The listing builds one solid part. Answer for the finished solid, in the listing's coordinates (mm). A direction names the side the tool comes from. Give positions to 0.01 mm unless a question says otherwise; leave off trailing zeros. Write each loop counter-clockwise with the first axis right and the second up, starting at its lowest first coordinate (ties: lowest second). Pieces come first, ordered by that corner, then holes. Notation, with made-up numbers: (49, 85.5) - (103, 85.5) arc R18 ccw to (103, 120.5) - close; hole circle Ø3 at (84, -38). An arc over 180 degrees is marked (long way). Return JSON: item names as keys, results as strings.
from build123d import *

# Parameters (mm, degrees)
SKETCH1_W           = 1524
SKETCH1_H           = 762
BOSS_EXTRUDE1_DEPTH = 1016
SKETCH3_W           = 762
SKETCH3_H           = 507.878356785
CUT_EXTRUDE1_DEPTH  = 1016
CUT_EXTRUDE2_DEPTH  = 260.604
SKETCH6_W           = 254
SKETCH6_H           = 507.878356785
CUT_EXTRUDE3_DEPTH  = 1081.278
SKETCH7_W           = 254
SKETCH7_H           = 508
CUT_EXTRUDE4_DEPTH  = 1081.278
SKETCH8_W           = 508.045957887
SKETCH8_H           = 254
CUT_EXTRUDE5_DEPTH  = 1081.278
CUT_EXTRUDE6_DEPTH  = 835.406


with BuildPart() as part:
    # Sketch1 → Boss-Extrude1 (new body)
    with BuildSketch(Plane.XY):
        with Locations((-762, 381)):
            Rectangle(SKETCH1_W, SKETCH1_H)
    extrude(amount=BOSS_EXTRUDE1_DEPTH)

    # Sketch3 → Cut-Extrude1 (cut)
    with BuildSketch(Plane(origin=(0, 0, 0), x_dir=(-1, 0, 0), z_dir=(0, 0, -1))):
        with Locations((1143, 508.060821607)):
            Rectangle(SKETCH3_W, SKETCH3_H)
    extrude(amount=-CUT_EXTRUDE1_DEPTH, mode=Mode.SUBTRACT)

    # Sketch5 → Cut-Extrude2 (cut)
    with BuildSketch(Plane(origin=(0, 254.121643215, 0), x_dir=(1, 0, 0), z_dir=(0, 1, 0))):
        Polygon((-1524, -1016), (-762, 0), (-1524, 0), align=None)
    extrude(amount=-CUT_EXTRUDE2_DEPTH, mode=Mode.SUBTRACT)

    # Sketch6 → Cut-Extrude3 (cut)
    with BuildSketch(Plane.ZY.offset(762)):
        with Locations((127, 508.060821607)):
            Rectangle(SKETCH6_W, SKETCH6_H)
    extrude(amount=-CUT_EXTRUDE3_DEPTH, mode=Mode.SUBTRACT)

    # Sketch7 → Cut-Extrude4 (cut)
    with BuildSketch(Plane.ZY.offset(762)):
        with Locations((381, 508.121643215)):
            Rectangle(SKETCH7_W, SKETCH7_H)
    extrude(amount=-CUT_EXTRUDE4_DEPTH, mode=Mode.SUBTRACT)

    # Sketch8 → Cut-Extrude5 (cut)
    with BuildSketch(Plane(origin=(0, 254.121643215, 0), x_dir=(1, 0, 0), z_dir=(0, 1, 0))):
        with Locations((-254.022978944, -127)):
            Rectangle(SKETCH8_W, SKETCH8_H)
    extrude(amount=-CUT_EXTRUDE5_DEPTH, mode=Mode.SUBTRACT)

    # Sketch10 → Cut-Extrude6 (cut)
    with BuildSketch(Plane.ZY.offset(762)):
        Polygon((1016, 762), (508, 762), (508, 508.060821608), align=None)
    extrude(amount=-CUT_EXTRUDE6_DEPTH, mode=Mode.SUBTRACT)


solid = part.part
Item 1: Consider L1, parallel to X at y = 261.5, z = 706.5; L2, parallel to Y at x = -1258, z = 961; L3, parallel to Z at x = -301.5, y = 451. Determine where each line is inside the solid, lowest interval first.
Answer below:
{"L1": "x = -762 to 0", "L2": "y = 0 to 254.12", "L3": "z = 508 to 1016"}
Item 2: For faces 1 (the face through (-603, 0, 614)), 2 (the face through (-508.046, 129, 129)), 3 (the face through (-386, 379, 508)), 4 (the face through (-762, 448, 758)), 5 (the face through (-637, 129, 0)), determine the directions among +Z, -Z, +X, -X, +Y, -Y from which every point of the face is accessible in a straight line to the end or side of a thin tool.
Answer below:
{"face 1": "+Z, -Z, +X, -X, -Y", "face 2": "-Z, +X, +Y, -Y", "face 3": "-Z, +X, -X, +Y", "face 4": "+Z, -Z, -X, +Y", "face 5": "-Z, +X, -X, +Y, -Y"}
Item 3: A cutting plane is placed at B-B on y = 61. Determine the outline of the cut face in (x, z), then the cut area to 3 significant figures.
Answer below:
{"outline": "(-1524, 1016) - (-762, 0) - (-508.05, 0) - (-508.05, 254) - (0, 254) - (0, 1016) - close", "area": "1,030,000 mm²"}
Item 4: Flat-ended cylindrical pins translate along their axes: P1, Ø2, axis at y = 136, z = 579, coming from the -X side; P2, Ø5, axis at x = -1124.5, z = 810, coming from the +Y side; P3, Ø10, axis at x = -303.5, y = 266.5, coming from the -Z side. Find the tip coordinate at first contact, or state that the pin passes through.
Answer below:
{"P1": "stops at x = -1197", "P2": "stops at y = 254.12", "P3": "stops at z = 508"}
Item 5: A cutting plane is placed at D-D on y = 338.5. Determine the outline of the cut face in (x, z).
Answer below:
{"outline": "(-762, 508) - (0, 508) - (0, 1016) - (-762, 1016) - close"}
Item 6: A cutting plane is placed at A-A on x = -142. Determine the outline of the cut face in (y, z).
Answer below:
{"outline": "(0, 254) - (254.12, 254) - (254.12, 508) - (508.06, 508) - (762, 1016) - (0, 1016) - close"}
Item 7: A cutting plane is placed at C-C on z = 418. Determine the outline of the cut face in (x, y).
Answer below:
{"outline": "(-1075.5, 0) - (0, 0) - (0, 254.12) - (-1075.5, 254.12) - close"}
